```python
from build123d import *

# Parameters (mm, degrees)
ESQUISSE1_W             = 50
ESQUISSE1_H             = 30
BOSS_EXTRU_1_DEPTH      = 30
ENL_V_MAT_EXTRU_1_REACH = 43.833
ESQUISSE2_R             = 6.35
CONG_1_R                = 10
ESQUISSE3_W             = 18
ESQUISSE3_H             = 30
ENL_V_MAT_EXTRU_2_DEPTH = 20


with BuildPart() as part:
    # Esquisse1 → Boss.-Extru.1 (new body)
    with BuildSketch(Plane.XY):
        Rectangle(ESQUISSE1_W, ESQUISSE1_H)
    extrude(amount=BOSS_EXTRU_1_DEPTH)

    # Esquisse2 → Enlèv. mat.-Extru.1 (cut, up to next)
    with BuildSketch(Plane.XY.offset(30), mode=Mode.PRIVATE) as enl_v_mat_extru_1_sk1:
        with Locations((-15, 0)):
            Circle(ESQUISSE2_R)
    enl_v_mat_extru_1_tool1 = extrude(enl_v_mat_extru_1_sk1.sketch, amount=-ENL_V_MAT_EXTRU_1_REACH, mode=Mode.PRIVATE) & part.part
    add(enl_v_mat_extru_1_tool1.solids().sort_by_distance((-15, 0, 30))[0], mode=Mode.SUBTRACT)

    # Congé1
    cong_1_edges = [part.edges().sort_by_distance(p)[0] for p in [
        (-25, -15, 15),
        (-25, 15, 15),
    ]]
    fillet(cong_1_edges, radius=CONG_1_R)

    # Esquisse3 → Enlèv. mat.-Extru.2 (cut)
    with BuildSketch(Plane.ZY.offset(25)):
        with Locations((15, 0)):
            Rectangle(ESQUISSE3_W, ESQUISSE3_H)
    extrude(amount=-ENL_V_MAT_EXTRU_2_DEPTH, mode=Mode.SUBTRACT)


solid = part.part
```
Work out the finished part from the listing and answer in its coordinate system (mm). A direction names the side the tool comes from. Give positions to 0.01 mm unless a question says otherwise; leave off trailing zeros. Loops run counter-clockwise (first coordinate to the right, second up) from the corner with the lowest first, then second, coordinate; pieces in that order, holes last. Notation, with made-up numbers: (65, 34) -> (114, 34) arc R27 ccw to (114, 71) -> close; hole circle Ø6 at (-29, 29.25). An arc over 180 degrees is marked (long way). Write item = value, one per line. Start each with the question number.
(1) The mould has two halves that part along X. Classify faces 1 (the flat face through (5, -15, 15)), 2 (the cylindrical face through (-21.344, 0.279, 27.042)), 3 (the cylindrical face through (-22.15, -11.99, 3.04)): +X half, -X half, draft (parallel to the pull), parting line (faces both ways), or undercut.
(2) Find section C-C on y = -10.5. Give the vertices of the cut face in (x, z).
(3) Given pin 1 Ø6 at (x, z) = (-19.5, 7.5) entering from +Y, flat-ended and moving along its own axis, determine where the tip first touches the part or whether it passes through.
(4) Find section A-A on z = 27.5. Give the vertices of the cut face in (x, y).
(5) Which of the six approach directions +Z, -Z, +X, -X, +Y, -Y give full straight-line access (tool end or side, diameter ignored) to faces 4 (the flat face through (-5, 0, 15)), 5 (the flat face through (-25, 0, 3))?
(6) Find the intervals of material crossed by probe 1 along Y at (x, z) = (-15, 28.2); probe 2 along Z at (x, y) = (-18, 8); probe 3 along X at (y, z) = (-9, 6.75), in increasing order. Write a range as from..to.
(7) Find section D-D on z = 16. Give the vertices of the cut face in (x, y).
(8) Find section B-B on y = 0. Give the vertices of the cut face in (x, z).
From the geometry:
q1.face_1 = draft
q1.face_2 = undercut
q1.face_3 = -X half
q2.outline = (-23.35, 0) -> (25, 0) -> (25, 30) -> (-23.35, 30) -> (-23.35, 24) -> (-5, 24) -> (-5, 6) -> (-23.35, 6) -> close
q3.pin_1 = 14.82
q4.outline = (-25, -5) arc R10 ccw to (-15, -15) -> (25, -15) -> (25, 15) -> (-15, 15) arc R10 ccw to (-25, 5) -> close; hole circle Ø12.7 at (-15, 0)
q5.face_4 = -X, +Y, -Y
q5.face_5 = +Z, -Z, -X, +Y, -Y
q6.probe_1 = -15..-6.35, 6.35..15
q6.probe_2 = 0..6, 24..30
q6.probe_3 = -5..25
q7.outline = (-5, -15) -> (25, -15) -> (25, 15) -> (-5, 15) -> close
q8.outline = (-25, 0) -> (-21.35, 0) -> (-21.35, 6) -> (-25, 6) -> close; (-25, 24) -> (-21.35, 24) -> (-21.35, 30) -> (-25, 30) -> close; (-8.65, 0) -> (25, 0) -> (25, 30) -> (-8.65, 30) -> (-8.65, 24) -> (-5, 24) -> (-5, 6) -> (-8.65, 6) -> close
